```python
from build123d import *

# Parameters (mm, degrees)
ESQUISSE2_R                         = 1.5
ENL_V_MAT_EXTRU_1_DEPTH             = 10
ESQUISSE3_R                         = 1.5
ENL_V_MAT_EXTRU_2_DEPTH             = 37.362755671
ENL_V_MAT_EXTRU_2_DIRECTION_2_REACH = 38.363
ESQUISSE4_R                         = 2.75
ENL_V_MAT_EXTRU_7_DEPTH             = 20
ENL_V_START                         = -8
ESQUISSE5_R                         = 8
ENL_V_MAT_EXTRU_8_DEPTH             = 8


with BuildPart() as part:
    # Esquisse1 → Révolution1 (revolve)
    with BuildSketch(Plane.XY):
        Polygon((8, 0), (8, 1.5), (14, 1.5), (14, 30.5), (8, 30.5), (8, 32), (2.5, 32), (2.5, 0), align=None)
    revolve(axis=Axis((0, 0, 0), (0, 1, 0)))

    # Esquisse2 → Enlèv. mat.-Extru.1 (cut)
    with BuildSketch(Plane(origin=(0, 30.5, 0), x_dir=(1, 0, 0), z_dir=(0, 1, 0))):
        with Locations(Location((0, 11, 0), (0, 0, 180))):
            Circle(ESQUISSE2_R)
        with Locations(Location((9.526279442, -5.5, 0), (0, 0, 180))):
            Circle(ESQUISSE2_R)
        with Locations(Location((-9.526279442, -5.5, 0), (0, 0, 180))):
            Circle(ESQUISSE2_R)
    extrude(amount=-ENL_V_MAT_EXTRU_1_DEPTH, mode=Mode.SUBTRACT)

    # Esquisse3 → Enlèv. mat.-Extru.2 (cut)
    with BuildSketch(Plane.XZ.offset(-1.5)):
        with Locations(Location((0, 5.5, 0), (0, 0, 180))):
            Circle(ESQUISSE3_R)
        with Locations(Location((4.763139721, -2.75, 0), (0, 0, 180))):
            Circle(ESQUISSE3_R)
        with Locations(Location((-4.763139721, -2.75, 0), (0, 0, 180))):
            Circle(ESQUISSE3_R)
    extrude(amount=-ENL_V_MAT_EXTRU_2_DEPTH, mode=Mode.SUBTRACT)

    # Esquisse3 → Enlèv. mat.-Extru.2 direction 2 (cut, up to next)
    with BuildSketch(Plane.XZ.offset(-1.5), mode=Mode.PRIVATE) as enl_v_mat_extru_2_direction_2_sk1:
        with Locations(Location((0, 5.5, 0), (0, 0, 180))):
            Circle(ESQUISSE3_R)
    enl_v_mat_extru_2_direction_2_tool1 = extrude(enl_v_mat_extru_2_direction_2_sk1.sketch, amount=ENL_V_MAT_EXTRU_2_DIRECTION_2_REACH, mode=Mode.PRIVATE) & part.part
    # Esquisse3 → Enlèv. mat.-Extru.2 direction 2 (cut, up to next)
    with BuildSketch(Plane.XZ.offset(-1.5), mode=Mode.PRIVATE) as enl_v_mat_extru_2_direction_2_sk2:
        with Locations(Location((4.763139721, -2.75, 0), (0, 0, 180))):
            Circle(ESQUISSE3_R)
    enl_v_mat_extru_2_direction_2_tool2 = extrude(enl_v_mat_extru_2_direction_2_sk2.sketch, amount=ENL_V_MAT_EXTRU_2_DIRECTION_2_REACH, mode=Mode.PRIVATE) & part.part
    # Esquisse3 → Enlèv. mat.-Extru.2 direction 2 (cut, up to next)
    with BuildSketch(Plane.XZ.offset(-1.5), mode=Mode.PRIVATE) as enl_v_mat_extru_2_direction_2_sk3:
        with Locations(Location((-4.763139721, -2.75, 0), (0, 0, 180))):
            Circle(ESQUISSE3_R)
    enl_v_mat_extru_2_direction_2_tool3 = extrude(enl_v_mat_extru_2_direction_2_sk3.sketch, amount=ENL_V_MAT_EXTRU_2_DIRECTION_2_REACH, mode=Mode.PRIVATE) & part.part
    add(enl_v_mat_extru_2_direction_2_tool1.solids().sort_by_distance((0, 1.5, 5.5))[0], mode=Mode.SUBTRACT)
    add(enl_v_mat_extru_2_direction_2_tool2.solids().sort_by_distance((4.76314, 1.5, -2.75))[0], mode=Mode.SUBTRACT)
    add(enl_v_mat_extru_2_direction_2_tool3.solids().sort_by_distance((-4.76314, 1.5, -2.75))[0], mode=Mode.SUBTRACT)

    # Esquisse4 → Enlèv. mat.-Extru.7 (cut)
    with BuildSketch(Plane.XZ.offset(-32)):
        with Locations(Location((0, 5.5, 0), (0, 0, 120.036983744))):
            Circle(ESQUISSE4_R)
        with Locations(Location((4.763139721, -2.75, 0), (0, 0, 299.963016256))):
            Circle(ESQUISSE4_R)
        with Locations(Location((-4.763139721, -2.75, 0), (0, 0, 179.963016256))):
            Circle(ESQUISSE4_R)
    extrude(amount=ENL_V_MAT_EXTRU_7_DEPTH, mode=Mode.SUBTRACT)

    # Esquisse5 → Enlèv. mat.-Extru.8 (cut)
    with BuildSketch(Plane.XZ.offset(ENL_V_START)):
        Circle(ESQUISSE5_R)
    extrude(amount=ENL_V_MAT_EXTRU_8_DEPTH, mode=Mode.SUBTRACT)


solid = part.part
```
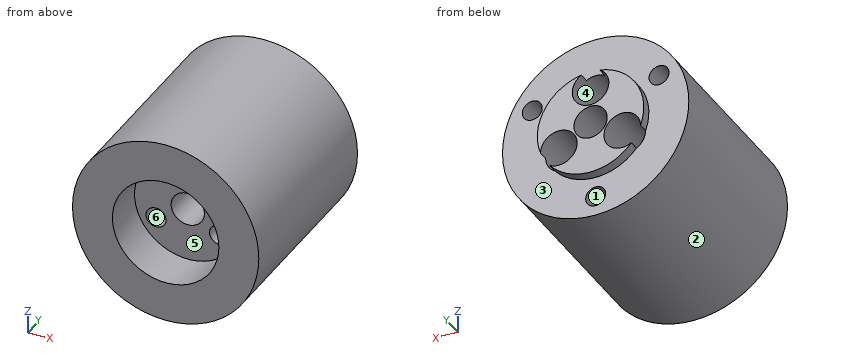
Input: part model. Units: mm. Frame: model coordinates. Face numbers are marked on the shaded views. A direction names the side the tool comes from. Coordinates: 2 decimals unless noted, no trailing zeros. Loops run counter-clockwise (first coordinate to the right, second up) from the corner with the lowest first, then second, coordinate; pieces in that order, holes last.
Q1. Section B-B, the plane y = 22.5. Return the cut outline in (x, z), and give its area (3 significant figures).
Results are:
outline: circle Ø28 at (0, 0); hole circle Ø3 at (-9.53, 5.5); hole circle Ø5.5 at (-4.76, -2.75); hole circle Ø5.5 at (0, 5.5); hole circle Ø5 at (0, 0); hole circle Ø3 at (0, -11); hole circle Ø5.5 at (4.76, -2.75); hole circle Ø3 at (9.53, 5.5)
area: 504 mm2
Q2. Section A-A, the plane x = 0. Return the cut outline in (y, z), and give its area (3 significant figures).
Results are:
outline: (1.5, -14) - (30.5, -14) - (30.5, -12.5) - (20.5, -12.5) - (20.5, -9.5) - (30.5, -9.5) - (30.5, -8) - (32, -8) - (32, -2.5) - (8, -2.5) - (8, -8) - (1.5, -8) - close; (1.5, 8) - (8, 8) - (8, 7) - (12, 7) - (12, 8.25) - (30.5, 8.25) - (30.5, 14) - (1.5, 14) - close; (8, 2.5) - (32, 2.5) - (32, 2.75) - (12, 2.75) - (12, 4) - (8, 4) - close
area: 460 mm2
Q3. Section D-D, the plane y = 10. Return the cut outline in (x, z).
Results are:
outline: circle Ø28 at (0, 0); hole circle Ø3 at (-4.76, -2.75); hole circle Ø5 at (0, 0); hole circle Ø3 at (0, 5.5); hole circle Ø3 at (4.76, -2.75)
Q4. Section C-C, the plane z = 5.5. Return the cut outline in (x, y), and give its area (3 significant figures).
Results are:
outline: (-12.87, 1.5) - (-5.81, 1.5) - (-5.81, 8) - (-1.5, 8) - (-1.5, 12) - (-2.75, 12) - (-2.75, 32) - (-5.81, 32) - (-5.81, 30.5) - (-8.03, 30.5) - (-8.03, 20.5) - (-11.03, 20.5) - (-11.03, 30.5) - (-12.87, 30.5) - close; (1.5, 8) - (5.81, 8) - (5.81, 1.5) - (12.87, 1.5) - (12.87, 30.5) - (11.03, 30.5) - (11.03, 20.5) - (8.03, 20.5) - (8.03, 30.5) - (5.81, 30.5) - (5.81, 32) - (2.75, 32) - (2.75, 12) - (1.5, 12) - close
area: 507 mm2
Q5. Contact query for flat-ended pins moving along their axis: pin 1 (1 mm diameter, centred on x = 7.5, z = 5.5, fed in from +Y); pin 2 (3.5 mm diameter, centred on x = 0, z = 5.5, fed in from +Y); pin 3 (2.5 mm diameter, centred on x = 0, z = -11, fed in from +Y). Output: stop coordinate, or through.
Results are:
pin 1: stops at y = 30.5
pin 2: stops at y = 12
pin 3: stops at y = 20.5
Q6. Mould query, pull axis X, two halves, no side actions, for the marked faces 1, 2 and 3. Classes: +X half, -X half, draft (parallel to the pull), parting line (faces both ways), or undercut.
Results are:
face 1: undercut
face 2: parting line
face 3: draft
Q7. Set-up query: the marked faces 4, 5 and 6. Return all of +Z, -Z, +X, -X, +Y, -Y with unobstructed straight access to the full face (end or side cutting, diameter ignored); none if empty.
Results are:
face 4: +Y
face 5: -Y
face 6: +Y, -Y
Q8. Line query: line 1 along X through (y, z) = (24.5, -3.75); line 2 along X through (y, z) = (21, -4.75); line 3 along Z through (x, y) = (2.25, 28.5). Output: solid intervals per line, ascending.
Results are:
line 1: x = -13.49 to -7.32, -2.2 to 2.2, 7.32 to 13.49
line 2: x = -13.17 to -6.65, -2.88 to 2.88, 6.65 to 13.17
line 3: z = -13.82 to -3.87, -1.63 to -1.09, 1.09 to 3.92, 7.08 to 13.82
